Autodesk Inventor part; units mm, degrees
ref_plane "YZ Plane" through (0, 0, 0) normal (1, 0, 0) x (0, 1, 0)
ref_plane "XZ Plane" through (0, 0, 0) normal (0, 1, 0) x (-1, 0, 0)
ref_plane "XY Plane" through (0, 0, 0) normal (0, 0, 1) x (1, 0, 0)
sketch "Sketch1" plane through (0, 0, 0) normal (0, 0, 1) x (1, 0, 0)
  circle A0 centre (0, 0) radius 2.6035
  line L0 (0.3297, 4.515) -> (1.8944, 4.515)
  line L1 (4.8382, 1.3026) -> (4.8382, -0.0642)
  line L2 (4.8382, -0.0642) -> (4.8382, -1.3419)
  line L3 (4.8382, -0.0642) -> (6.1159, -0.0642) construction
  line L4 (1.6632, -4.5854) -> (0, -4.5854)
  line L5 (0, -4.5854) -> (-1.4104, -4.5854)
  line L6 (-4.5212, -1.3462) -> (-4.5212, 0)
  line L7 (-4.5212, 0) -> (-4.5212, 1.3026)
  line L8 (-1.0165, 4.515) -> (0.3297, 4.515)
  line L9 (1.8944, 4.515) -> (10.2327, 4.515) construction
  line L10 (1.8944, 4.515) -> (4.6655, 7.2861)
  line L11 (1.8944, 4.515) -> (5.8133, 4.515) construction
  line L12 (4.8382, 1.3026) -> (7.6093, 4.0737)
  line L13 (-1.0165, 4.515) -> (-3.7876, 7.2861)
  line L14 (-4.5212, 1.3026) -> (-7.2923, 4.0737)
  line L15 (-4.5212, -1.3462) -> (-7.2923, -4.1173)
  line L16 (-1.4104, -4.5854) -> (-4.1173, -7.2923)
  line L17 (1.6632, -4.5854) -> (4.4343, -7.3565)
  line L18 (4.8382, -1.3419) -> (7.6093, -4.113)
  line L19 (4.8382, -1.3419) -> (8.7572, -1.3419) construction
  line L20 (-2.8896, 9.4541) -> (-1.7646, 9.4541)
  line L21 (3.7675, 9.4541) -> (2.6425, 9.4541)
  line L22 (-9.4603, 3.1757) -> (-9.4603, 2.0507)
  line L23 (-9.4603, -3.2193) -> (-9.4603, -2.0943)
  line L24 (-3.2193, -9.4603) -> (-2.0943, -9.4603)
  line L25 (3.5363, -9.5246) -> (2.4114, -9.5246)
  line L26 (9.7774, -3.215) -> (9.7774, -2.0901)
  line L27 (9.7774, 3.1757) -> (9.7774, 2.0507)
  line L28 (-1.7646, 9.4541) -> (-1.7646, 12.6291)
  line L29 (-9.4603, 2.0507) -> (-12.6353, 2.0507)
  line L30 (-9.4603, -2.0943) -> (-12.6353, -2.0943)
  line L31 (-2.0943, -9.4603) -> (-2.0943, -12.6353)
  line L32 (2.4114, -9.5246) -> (2.4114, -12.6996)
  line L33 (9.7774, -2.0901) -> (12.9524, -2.0901)
  line L34 (9.7774, 2.0507) -> (12.9524, 2.0507)
  line L35 (2.6425, 9.4541) -> (2.6425, 12.6291)
  line L36 (-1.7646, 12.6291) -> (-9.4603, 12.6291)
  line L37 (-12.6353, 9.4541) -> (-12.6353, 2.0507)
  line L38 (-12.6353, -2.0943) -> (-12.6353, -11.3653)
  line L39 (-11.3653, -12.6353) -> (-2.0943, -12.6353)
  line L40 (12.9524, -2.0901) -> (12.9524, -11.4296)
  line L41 (11.6824, -12.6996) -> (2.4114, -12.6996)
  line L42 (12.9524, 2.0507) -> (12.9524, 11.3591)
  line L43 (11.6824, 12.6291) -> (2.6425, 12.6291)
  arc A1 (-9.4603, 12.6291) -> (-12.6353, 9.4541) centre (-9.4603, 9.4541) ccw
  arc A2 (-2.8896, 9.4541) -> (-3.7876, 7.2861) centre (-2.8896, 8.1841) ccw
  arc A3 (-7.2923, 4.0737) -> (-9.4603, 3.1757) centre (-8.1903, 3.1757) ccw
  arc A4 (-9.4603, -3.2193) -> (-7.2923, -4.1173) centre (-8.1903, -3.2193) ccw
  arc A5 (-4.1173, -7.2923) -> (-3.2193, -9.4603) centre (-3.2193, -8.1903) ccw
  arc A6 (3.5363, -9.5246) -> (4.4343, -7.3565) centre (3.5363, -8.2546) ccw
  arc A7 (7.6093, -4.113) -> (9.7774, -3.215) centre (8.5074, -3.215) ccw
  arc A8 (9.7774, 3.1757) -> (7.6093, 4.0737) centre (8.5074, 3.1757) ccw
  arc A9 (4.6655, 7.2861) -> (3.7675, 9.4541) centre (3.7675, 8.1841) ccw
  arc A10 (12.9524, 11.3591) -> (11.6824, 12.6291) centre (11.6824, 11.3591) ccw
  arc A11 (11.6824, -12.6996) -> (12.9524, -11.4296) centre (11.6824, -11.4296) ccw
  arc A12 (-12.6353, -11.3653) -> (-11.3653, -12.6353) centre (-11.3653, -11.3653) ccw
  point P0 (4.8382, 4.515)
  point P1 (4.8382, -4.5854)
  point P2 (-4.5212, -4.5854)
  point P3 (-4.5212, 4.515)
  point P4 (6.8335, 9.4541)
  point P5 (9.7774, 6.2417)
  point P6 (-5.9556, 9.4541)
  point P7 (-9.4603, 6.2417)
  point P8 (-9.4603, -6.2853)
  point P9 (-6.2853, -9.4603)
  point P10 (6.6024, -9.5246)
  point P11 (9.7774, -6.2811)
  dimension "d0" = 5.207
  dimension "d1" = 4.5085
  dimension "d2" = 90
  dimension "d3" = 4.5212
  dimension "d4" = 90
  dimension "d5" = 4.5212
  dimension "d9" = 6.985
  dimension "d10" = 45
  dimension "d11" = 6.985
  dimension "d12" = 6.985
  dimension "d13" = 6.985
  dimension "d14" = 6.985
  dimension "d15" = 6.985
  dimension "d16" = 6.985
  dimension "d17" = 45
  dimension "d18" = 4.191
  dimension "d19" = 4.191
  dimension "d20" = 4.191
  dimension "d21" = 4.191
  dimension "d22" = 4.191
  dimension "d23" = 4.191
  dimension "d24" = 4.191
  dimension "d25" = 4.191
  dimension "d26" = 3.175
  dimension "d27" = 3.175
  dimension "d28" = 3.175
  dimension "d29" = 3.175
  dimension "d30" = 3.175
  dimension "d31" = 1.27
  dimension "d32" = 1.27
extrude "Extrusion1" add sketch "Sketch1" along normal blind 25.4
properties part number "kylestslot"
Read the model definition and answer for the solid it produces. Units are mm, in the model's axes. A direction names the side the tool comes from. Give positions to 0.01 mm unless a question says otherwise; leave off trailing zeros. Write each loop counter-clockwise with the first axis right and the second up, starting at its lowest first coordinate (ties: lowest second). Pieces come first, ordered by that corner, then holes. Notation, with made-up numbers: (-23, 52.5) - (19, 52.5) arc R12 ccw to (19, 66.5) - close; hole circle Ø6 at (-29, 51). An arc over 180 degrees is marked (long way). Write item = value, one per line. Start each with the question number.
Item 1: Find section A-A (x = 10.25). Give the vertices of the cut face in (y, z).
Item 2: Find the intervals of material crossed by probe 1 along Y at (x, z) = (0, 18.5) (1 decimal); probe 2 along X at (y, z) = (-10.25, 17); probe 3 along Y at (x, z) = (11, 3.5), in increasing order. Write a range as [from, to].
Item 3: The mould has two halves that part along Y. Classify faces 1 (the cylindrical face through (12.59, -12.32, 12.52)), 2 (the flat face through (4.838, 0, 13)), 3 (the flat face through (0, -3, 0)): +Y half, -Y half, draft (parallel to the pull), parting line (faces both ways), or undercut.
Item 4: A tool of negligible diameter and unlimited length cuts with its end or side. For faces 4 (the flat face through (-11, 2.051, 13)), 5 (the flat face through (11, 2.051, 13)), 6 (the flat face through (3, 9.454, 13)), from which of +Z, -Z, +X, -X, +Y, -Y can it reach the whole face along a straight path? Write none if from no direction.
Item 5: Each of these flat-tipped pins is pushed along its axis until it touches: P1, Ø12, axis at x = 6.5, y = -7.5, coming from the -Z side; P2, Ø2.5, axis at x = 0.5, z = 10.5, coming from the -Y side; P3, Ø10, axis at x = -8, z = 6.5, coming from the -Y side; P4, Ø1.5, axis at x = 1, z = 18, coming from the +Y side (3 decimals). Where does it stop, or does it pass through?
Item 6: Find section B-B (y = 0). Give the vertices of the cut face in (x, z).
Response:
q1.outline = (-12.7, 0) - (-2.09, 0) - (-2.09, 25.4) - (-12.7, 25.4) - close; (2.05, 0) - (12.63, 0) - (12.63, 25.4) - (2.05, 25.4) - close
q2.probe_1 = [-4.6, -2.6], [2.6, 4.5]
q2.probe_2 = [-12.64, -2.09], [2.41, 12.95]
q2.probe_3 = [-12.7, -2.09], [2.05, 12.63]
q3.face_1 = -Y half
q3.face_2 = undercut
q3.face_3 = draft
q4.face_4 = +Z, -Z, -X
q4.face_5 = +Z, -Z, +X
q4.face_6 = +Z, -Z
q5.P1 = 0
q5.P2 = -4.67
q5.P3 = -12.64
q5.P4 = 4.515
q6.outline = (-4.52, 0) - (-2.6, 0) - (-2.6, 25.4) - (-4.52, 25.4) - close; (2.6, 0) - (4.84, 0) - (4.84, 25.4) - (2.6, 25.4) - close
